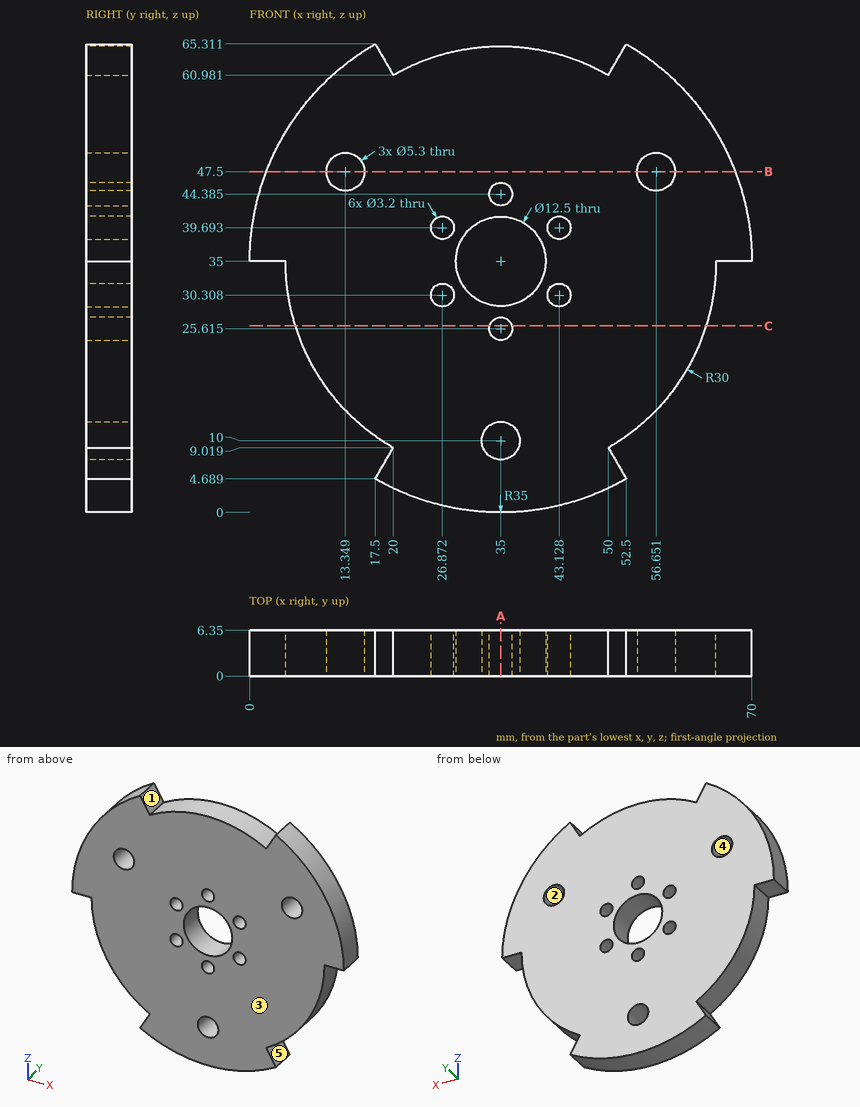
For this review, use the dimensioned drawing (mm, ordinates from the lowest corner) and the shaded views. A direction names the side the tool comes from. Give positions to 0.01 mm unless a question says otherwise; leave off trailing zeros. Write each loop counter-clockwise with the first axis right and the second up, starting at its lowest first coordinate (ties: lowest second). Pieces come first, ordered by that corner, then holes. Notation, with made-up numbers: M 47.25,83 L 73.25,83 A15 ccw 73.25,103 Z; hole C 46.25,62.5 d9. An arc over 180 degrees is marked long. Write item = value, one per line. Start each with the question number.
Q1. Clearance check with flat-ended pins moving along their axes: pin 1 (3 mm diameter, centred on y = 2.5, z = 41.5, fed in from -X); pin 2 (8 mm diameter, centred on x = 16, z = 12, fed in from -Y). State where each tip first meets the part, or that it passes through.
Q2. We need section C-C (z = 26). State the section outline as (x, y) points, plus the area to 3 significant figures.
Q3. We need section B-B (z = 47.5). State the section outline as (x, y) points.
Q4. Mouldability with a two-part tool opening along X and no side actions: class the marked faces 3, 4 and 5 as released by +X, released by -X, zero draft, split by the parting line, or undercut.
Q5. Machinability: for the marked faces 1 and 2, which of the approach directions +Z, -Z, +X, -X, +Y, -Y give a long, thin tool a straight path to every point of the face, cutting with its end or side? Answer none if there is none.
Q6. For line 1 (X direction, y = 1.5, z = 30.5) (1 decimal); line 2 (X direction, y = 3.25, z = 47.5); line 3 (Z direction, x = 42.5, y = 1) (1 decimal), list the stretches that pass through material, from the lowest coordinate up.
Q7. We need section A-A (x = 35). Give the number of separate pieces and of enclosed holes in the cut face, plus the area to 3 significant figures.
Result set:
q1.pin_1 = 0.36
q1.pin_2 = 0
q2.outline = M 6.38,0 L 33.45,0 L 33.45,6.35 L 6.38,6.35 Z; M 36.55,0 L 63.62,0 L 63.62,6.35 L 36.55,6.35 Z
q2.area = 344 mm2
q3.outline = M 2.31,0 L 10.7,0 L 10.7,6.35 L 2.31,6.35 Z; M 16,0 L 54,0 L 54,6.35 L 16,6.35 Z; M 59.3,0 L 67.69,0 L 67.69,6.35 L 59.3,6.35 Z
q4.face_3 = zero draft
q4.face_4 = undercut
q4.face_5 = released by +X
q5.face_1 = +Z, +Y, -Y
q5.face_2 = +Y, -Y
q6.line_1 = 5.3 to 25.3, 28.5 to 30.7, 39.3 to 41.5, 44.7 to 64.7
q6.line_2 = 2.31 to 10.7, 16 to 54, 59.3 to 67.69
q6.line_3 = 0.8 to 28.8, 31.8 to 38.2, 41.2 to 64
q7.separate_pieces = 5
q7.enclosed_holes = 0
q7.area = 259 mm2
